Source: CAD feature listing. Evaluate the final solid. Frame: model axes, mm. A direction names the side the tool comes from. Give positions to 0.01 mm unless a question says otherwise; leave off trailing zeros. Order: outer loops, then holes, each group sorted by start corner. A loop starts at its lowest first (then second) coordinate and runs counter-clockwise, first axis right, second up. Notation, with made-up numbers: M -10,46.25 L 8,46.25 A23 ccw 8,74.25 Z; hole C 67,52 d10. An arc over 180 degrees is marked long. One line per question, with ' | ' between items. Start each with the question number.
Solid Edge part; units mm, degrees
sketch "Sketch1" plane through (0, 0, 0) normal (0, 0, 1) x (1, 0, 0)
  circle A0 centre (0, 0) radius 35
extrude "Protrusion1" add sketch "Sketch1" along normal blind 63
sketch "Sketch2" plane through (0, 0, 63) normal (0, 0, 1) x (1, 0, 0)
  line L0 (-10.5, 10.25) -> (30, 10.25)
  line L1 (30, 10.25) -> (30, -10.25)
  line L2 (30, -10.25) -> (-10.5, -10.25)
  line L3 (-10.5, -10.25) -> (-10.5, 10.25)
  dimension "D1" = 10.5
  dimension "D2" = 10.5
extrude "Extrusionsausschnitt_1" cut sketch "Sketch2" against normal blind 45
sketch "Sketch3" plane through (0, 0, 0) normal (0, 0, -1) x (1, 0, 0)
  circle A0 centre (0, 0) radius 6.5
extrude "Extrusionsausschnitt_4" cut sketch "Sketch3" against normal blind 9
sketch "Sketch4" plane through (0, 0, 0) normal (0, 0, -1) x (1, 0, 0)
  line L0 (-0.5109, 6.4799) -> (-18.0109, 5.1)
  line L1 (-18.0109, 5.1) -> (-18.0109, -5.1)
  line L2 (-18.0109, -5.1) -> (-0.5109, -6.4799)
  line L3 (-0.5109, -6.4799) -> (-0.5109, 6.4799)
  dimension "D1" = 18.0109
extrude "Cutout1" cut sketch "Sketch4" against normal up to vertex (9 mm away)
sketch "Sketch5" plane through (0, 0, 63) normal (0, 0, 1) x (1, 0, 0)
  circle A0 centre (0, 0) radius 7.5
extrude "Extrusionsausschnitt_6" cut sketch "Sketch5" against normal blind 51
sketch "Sketch6" plane through (0, 0, 0) normal (0, 0, -1) x (1, 0, 0)
  circle A0 centre (0, 0) radius 4
extrude "Cutout2" cut sketch "Sketch6" against normal through all
sketch "Sketch7" plane through (9.75, 10.25, 41.5) normal (0, -1, 0) x (1, 0, 0)
  line L0 (20.25, -23.5) -> (20.25, 21.5)
  line L1 (20.25, 21.5) -> (-20.25, 21.5)
  line L2 (-20.25, 21.5) -> (-20.25, -23.5)
  line L3 (-20.25, -23.5) -> (20.25, -23.5)
extrude "Cutout3" cut sketch "Sketch7" against normal through all
sketch "Sketch8" plane through (9.75, -10.25, 41.5) normal (0, 1, 0) x (-1, 0, 0)
  line L0 (-20.25, 21.5) -> (-0.25, 21.5)
  line L1 (-0.25, 21.5) -> (-0.25, 16.5)
  line L2 (-0.25, 16.5) -> (-20.25, 16.5)
  line L3 (-20.25, 16.5) -> (-20.25, 21.5)
  dimension "D1" = 20.25
  dimension "D2" = 0.25
extrude "Protrusion2" add sketch "Sketch8" along normal up to vertex (28.2778 mm away)
sketch "Sketch9" plane through (-13, 4, 41.5) normal (0, -1, 0) x (0, 0, 1)
  line L0 (-13.5, 2.5) -> (-23.5, 2.5)
  line L1 (-23.5, 2.5) -> (-23.5, -2.5)
  line L2 (-13.5, -2.5) -> (-23.5, -2.5)
  line L3 (-13.5, 2.5) -> (-13.5, -2.5)
  dimension "D1" = 13.5
extrude "Cutout4" cut sketch "Sketch9" against normal through all
sketch "Sketch10" plane through (-13, 4, 25) normal (0, 1, 0) x (-1, 0, 0)
  line L0 (-2.5, 3) -> (12.5, 3)
  line L1 (12.5, 3) -> (12.5, -7)
  line L2 (12.5, -7) -> (-2.5, -7)
  line L3 (-2.5, -7) -> (-2.5, 3)
  dimension "D1" = 2.5
extrude "Cutout5" cut sketch "Sketch10" along normal through all and the other way up to vertex (14.25 mm away)
chamfer "Fase_1" distance 3 angle 45 1 edges at (-35, 0, 0)
Item 1: Pin query (flat end, axial travel): pin 1 Ø1 at (y, z) = (-10.5, 14) entering from +X; pin 2 Ø2.5 at (y, z) = (6, 61.5) entering from -X; pin 3 Ø5 at (y, z) = (1.5, 21) entering from +X; pin 4 Ø12 at (x, y) = (-2, 1.5) entering from +Z. Return the tip coordinate at first contact, or that it passes through.
Item 2: Line query: line 1 (Y direction, x = 0, z = 14); line 2 (X direction, y = 0, z = 9.8); line 3 (Z direction, x = -22, y = 19). Output: solid intervals per line, ascending.
Item 3: Cut plane A-A on y = 0. Return the cut outline in (x, z), and give its area (3 significant figures).
Item 4: Mould query, pull axis X, two halves, no side actions, for faces 6 (the cylindrical face through (-0.867, 3.905, 10.479)), 7 (the flat face through (3, -3, 12)), 8 (the flat face through (0, -16, 63)), 9 (the cylindrical face through (-4.56, -34.7, 32.58)). Classes: pulls with the +X half, pulls with the -X half, needs draft (parallel to the pull), parting line crosses it, or undercut.
Item 5: Cut plane C-C on z = 29. Return the cut outline in (x, y), and give its area (3 significant figures).
Item 6: Reachability of faces 1 (the flat face through (10, 4, 61)), 2 (the flat face through (-9.14, -5.8, 4.44)), 3 (the flat face through (20, 18.028, 61)), 4 (the flat face through (20, 4, 58)), 5 (the cylindrical face through (-7.493, 0.33, 15.042)) from +Z, -Z, +X, -X, +Y, -Y: full face, straight path, thin tool, end or side. Return the list, or none.
Results are:
1) pin 1: stops at x = 33.54 | pin 2: stops at x = -34.68 | pin 3: stops at x = 35 | pin 4: stops at z = 18
2) line 1: y = -35 to -7.5, 7.5 to 35 | line 2: x = -35 to -4, 4 to 35 | line 3: z = 0 to 18, 28 to 63
3) outline: M -35,3 L -32,0 L -18.01,0 L -18.01,9 L -4,9 L -4,12 L -7.5,12 L -7.5,18 L -25.5,18 L -25.5,28 L -10.5,28 L -10.5,63 L -35,63 Z; M 4,9 L 6.5,9 L 6.5,0 L 32,0 L 35,3 L 35,63 L 10,63 L 10,58 L 30,58 L 30,18 L 7.5,18 L 7.5,12 L 4,12 Z | area: 2,190 mm2
4) face 6: undercut | face 7: undercut | face 8: needs draft | face 9: parting line crosses it
5) outline: M -10.5,-10.25 L -10.5,33.39 A35 ccw long 30,18.03 L 30,-10.25 Z | area: 2,170 mm2
6) face 1: +Z, +Y | face 2: -Z | face 3: +Z, +X, +Y | face 4: +Y | face 5: +Z
